Source: CAD feature listing. Evaluate the final solid. Frame: model axes, mm. A direction names the side the tool comes from. Round coordinates to 2 decimals unless told otherwise and drop trailing zeros. Write each loop counter-clockwise with the first axis right and the second up, starting at its lowest first coordinate (ties: lowest second). Pieces come first, ordered by that corner, then holes. Notation, with made-up numbers: (-29.5, 73) -> (-4.5, 73) arc R24 cw to (-4.5, 86) -> close; hole circle Ø1 at (42, 85). An arc over 180 degrees is marked (long way). Return JSON: item names as keys, results as strings. Group by question number.
from build123d import *

# Parameters (mm, degrees)
SKETCH1_W           = 28.9
SKETCH1_H           = 19.9
SKETCH1_W_2         = 26.9
SKETCH1_H_2         = 17.9
BOSS_EXTRUDE1_DEPTH = 15
SKETCH1_3_W         = 28.9
SKETCH1_3_H         = 19.9
SKETCH1_3_W_2       = 26.9
SKETCH1_3_H_2       = 17.9
SKETCH1_3_W_3       = 26.5
SKETCH1_3_H_3       = 17.5
BOSS_EXTRUDE2_DEPTH = 4
SKETCH2_R           = 2.5
BOSS_EXTRUDE3_DEPTH = 4
FILLET1_R           = 0.4
FILLET2_R           = 0.4


with BuildPart() as part:
    # Sketch1 → Boss-Extrude1 (new body)
    with BuildSketch(Plane(origin=(0, 0, 0), x_dir=(1, 0, 0), z_dir=(0, 1, 0))):
        with Locations((13.25, 8.75)):
            Rectangle(SKETCH1_W, SKETCH1_H)
        with Locations((13.25, 8.75)):
            Rectangle(SKETCH1_W_2, SKETCH1_H_2, mode=Mode.SUBTRACT)
    extrude(amount=BOSS_EXTRUDE1_DEPTH)

    # Sketch1_3 → Boss-Extrude2 (add)
    # profile 1 of 3: a face of its own
    with BuildSketch(Plane(origin=(0, 0, 0), x_dir=(1, 0, 0), z_dir=(0, 1, 0))):
        with Locations((13.25, 8.75)):
            Rectangle(SKETCH1_3_W, SKETCH1_3_H)
        with Locations((13.25, 8.75)):
            Rectangle(SKETCH1_3_W_2, SKETCH1_3_H_2, mode=Mode.SUBTRACT)
    # profile 2 of 3: a face of its own
    with BuildSketch(Plane(origin=(0, 0, 0), x_dir=(1, 0, 0), z_dir=(0, 1, 0))):
        with Locations((13.25, 8.75)):
            Rectangle(SKETCH1_3_W_2, SKETCH1_3_H_2)
        with Locations((13.25, 8.75)):
            Rectangle(SKETCH1_3_W_3, SKETCH1_3_H_3, mode=Mode.SUBTRACT)
    # profile 3 of 3: a face of its own
    with BuildSketch(Plane(origin=(0, 0, 0), x_dir=(1, 0, 0), z_dir=(0, 1, 0))):
        with Locations((13.25, 8.75)):
            Rectangle(SKETCH1_3_W_3, SKETCH1_3_H_3)
    extrude(amount=-BOSS_EXTRUDE2_DEPTH)

    # Sketch2 → Boss-Extrude3 (add)
    with BuildSketch(Plane.XZ.offset(4)):
        with Locations(Location((8.25, -3.8, 0), (0, 0, 90))):
            Circle(SKETCH2_R)
        with Locations(Location((18.25, -3.8, 0), (0, 0, 90))):
            Circle(SKETCH2_R)
    extrude(amount=BOSS_EXTRUDE3_DEPTH)

    # Fillet1
    fillet1_edges = [part.edges().sort_by_distance(p)[0] for p in [
        (27.7, -4, -8.75),
        (13.25, -4, 1.2),
        (-1.2, -4, -8.75),
        (13.25, -4, -18.7),
        (8.25, -4, -6.3),
        (8.25, -8, -6.3),
        (18.25, -4, -6.3),
        (18.25, -8, -6.3),
    ]]
    fillet(fillet1_edges, radius=FILLET1_R)

    # Fillet2
    fillet2_edges = [part.edges().sort_by_distance(p)[0] for p in [
        (26.7, 7.5, 0.2),
        (26.7, 7.5, -17.7),
        (-0.2, 7.5, -17.7),
        (-0.2, 7.5, 0.2),
    ]]
    fillet(fillet2_edges, radius=FILLET2_R)


solid = part.part
Item 1: Cut plane C-C on y = -6. Output: boundary loops of the cut face in (x, z).
Item 2: First-contact query: pin 1 Ø5 at (x, z) = (15.5, -12) entering from -Y; pin 2 Ø9 at (x, z) = (7, -5.5) entering from +Y. Flat tips, straight axial feed; report the tip coordinate or a pass-through.
Item 3: Material intervals for probe 1 along X at (y, z) = (5.5, -16.25); probe 2 along Z at (x, y) = (13.5, 7.25); probe 3 along Y at (x, z) = (8.75, -7.25), sorted ascending.
Item 4: Cut plane B-B on x = 8.25. Output: boundary loops of the cut face in (y, z), and give its area (3 significant figures).
Item 5: Pull-direction query (X, two-part tool) for faces 4 (the flat face through (18, -8, -4)), 5 (the flat face through (13, 0, -9)), 6 (the flat face through (-0.2, 7, -9)), 7 (the flat face through (27.7, 6, -9)); classes: +X half, -X half, draft (parallel to the pull), parting line (faces both ways), or undercut.
Item 6: Cut plane A-A on y = 12. Output: boundary loops of the cut face in (x, z), and give its area (3 significant figures).
Item 7: Cut plane D-D on z = -3.8. Output: boundary loops of the cut face in (x, y).
Item 8: Set-up query: faces 1 (the flat face through (13, 7, 0.2)), 2 (the cylindrical face through (10.7, -6, -4.3)), 3 (the flat face through (12, 15, 1)). Return all of +Z, -Z, +X, -X, +Y, -Y with unobstructed straight access to the full face (end or side cutting, diameter ignored); none if empty.
Here are the results:
{
 "1": {"outline": "circle Ø5 at (8.25, -3.8); circle Ø5 at (18.25, -3.8)"},
 "2": {"pin 1": "stops at y = -4", "pin 2": "stops at y = 0"},
 "3": {"probe 1": "x = -1.2 to -0.2, 26.7 to 27.7", "probe 2": "z = -18.7 to -17.7, 0.2 to 1.2", "probe 3": "y = -4 to 0"},
 "4": {"outline": "(-8, -5.9) arc R0.4 ccw to (-7.6, -6.3) -> (-4.4, -6.3) arc R0.4 cw to (-4, -6.7) -> (-4, -18.3) arc R0.4 ccw to (-3.6, -18.7) -> (15, -18.7) -> (15, -17.7) -> (0, -17.7) -> (0, 0.2) -> (15, 0.2) -> (15, 1.2) -> (-3.6, 1.2) arc R0.4 ccw to (-4, 0.8) -> (-4, -0.9) arc R0.4 cw to (-4.4, -1.3) -> (-7.6, -1.3) arc R0.4 ccw to (-8, -1.7) -> close", "area": "130 mm^2"},
 "5": {"face 4": "draft", "face 5": "undercut", "face 6": "undercut", "face 7": "+X half"},
 "6": {"outline": "(-1.2, -18.7) -> (27.7, -18.7) -> (27.7, 1.2) -> (-1.2, 1.2) -> close; hole (-0.2, -17.3) arc R0.4 ccw to (0.2, -17.7) -> (26.3, -17.7) arc R0.4 ccw to (26.7, -17.3) -> (26.7, -0.2) arc R0.4 ccw to (26.3, 0.2) -> (0.2, 0.2) arc R0.4 ccw to (-0.2, -0.2) -> close", "area": "93.7 mm^2"},
 "7": {"outline": "(-1.2, -3.6) arc R0.4 ccw to (-0.8, -4) -> (5.35, -4) arc R0.4 cw to (5.75, -4.4) -> (5.75, -7.6) arc R0.4 ccw to (6.15, -8) -> (10.35, -8) arc R0.4 ccw to (10.75, -7.6) -> (10.75, -4.4) arc R0.4 cw to (11.15, -4) -> (15.35, -4) arc R0.4 cw to (15.75, -4.4) -> (15.75, -7.6) arc R0.4 ccw to (16.15, -8) -> (20.35, -8) arc R0.4 ccw to (20.75, -7.6) -> (20.75, -4.4) arc R0.4 cw to (21.15, -4) -> (27.3, -4) arc R0.4 ccw to (27.7, -3.6) -> (27.7, 15) -> (26.7, 15) -> (26.7, 0) -> (-0.2, 0) -> (-0.2, 15) -> (-1.2, 15) -> close"},
 "8": {"face 1": "+Y", "face 2": "-Y", "face 3": "+Z, -Z, +X, -X, +Y"}
}
